Here's how the part is built. I have some questions about the finished solid (model axes, mm). Give positions to 0.01 mm unless a question says otherwise; leave off trailing zeros. Write each loop counter-clockwise with the first axis right and the second up, starting at its lowest first coordinate (ties: lowest second). Pieces come first, ordered by that corner, then holes. Notation, with made-up numbers: (-12, -34) -> (40, -34) arc R33 cw to (40, -2) -> close; hole circle Ø3 at (41.25, 58.25). An arc over 180 degrees is marked (long way). Answer as CSV lines item,"result". Start each with the question number.
Solid Edge part; units mm, degrees
sketch "Sketch1" plane through (0, 0, 0) normal (0, 0, 1) x (1, 0, 0)
  line L0 (-15, -15) -> (15, -15)
  line L1 (15, -15) -> (15, 15)
  line L2 (15, 15) -> (-15, 15)
  line L3 (-15, 15) -> (-15, -15)
extrude "Protrusion1" add sketch "Sketch1" along normal blind 500
sketch "Sketch2" plane through (-15, 0, 250) normal (-1, 0, 0) x (0, 0, -1)
  line L0 (230, 3.5) -> (110, 3.5)
  line L1 (110, 3.5) -> (110, -3.5)
  line L2 (110, -3.5) -> (230, -3.5)
  line L3 (230, -3.5) -> (230, 3.5)
extrude "Extrusionsausschnitt_5" cut sketch "Sketch2" against normal blind 310
fillet "Verrundung_1" radius 3.5 4 edges at (0, 3.5, 140) (0, -3.5, 140) (0, 3.5, 20) (0, -3.5, 20)
mirror "Mirror1" about plane through (0, 0, 250) normal (0, 0, -1) of "Extrusionsausschnitt_5", "Verrundung_1"
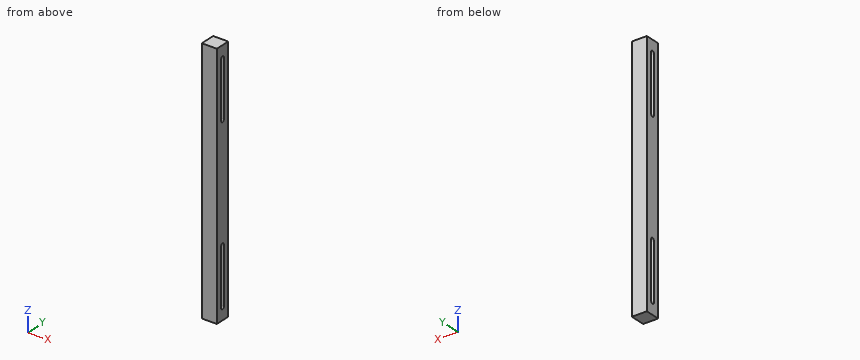
Item 1: If we section it at B-B (x = 6.5): State how many separate pieces and enclosed holes the cut face has, and give its area (3 significant figures).
Item 2: If I drill on line 1 (Z direction, x = 9.5, y = 0.5); line 2 (Y direction, x = -12.25, z = 425); line 3 (Z direction, x = -7.75, y = 2.5), over which ranges is the centre line in solid material (lowest first)? Write a range as [from, to].
Item 3: I'm going to push a flat-ended pin straight in: pin 1 (2 mm diameter, centred on x = -7, y = 7.5, fed in from -Z). Where does the tip first touch, or does it pass through?
Item 4: If we section it at A-A (z = 446): Please give me the cut outline in (x, y).
Final values:
1,separate pieces,"1"
1,enclosed holes,"2"
1,area,"13,300 mm2"
2,line 1,"[0, 20.04], [139.96, 360.04], [479.96, 500]"
2,line 2,"[-15, -3.5], [3.5, 15]"
2,line 3,"[0, 21.05], [138.95, 361.05], [478.95, 500]"
3,pin 1,"z = 0"
4,outline,"(-15, -15) -> (15, -15) -> (15, -3.5) -> (-15, -3.5) -> close; (-15, 3.5) -> (15, 3.5) -> (15, 15) -> (-15, 15) -> close"
